from build123d import *

# Parameters (mm, degrees)
CROQUIS2_R              = 83.82
CROQUIS2_R_2            = 80.01
SALIENTE_EXTRUIR1_DEPTH = 81.28
CROQUIS4_R              = 80.01
CROQUIS4_R_2            = 76.454
SALIENTE_EXTRUIR2_DEPTH = 4.572


with BuildPart() as part:
    # Croquis2 → Saliente-Extruir1 (new body)
    with BuildSketch(Plane(origin=(0, 0, 0), x_dir=(1, 0, 0), z_dir=(0, 1, 0))):
        with Locations(Location((0, 0, 0), (0, 0, 270))):
            Circle(CROQUIS2_R)
        with Locations(Location((0, 0, 0), (0, 0, 270))):
            Circle(CROQUIS2_R_2, mode=Mode.SUBTRACT)
    extrude(amount=-SALIENTE_EXTRUIR1_DEPTH)

    # Croquis4 → Saliente-Extruir2 (add)
    with BuildSketch(Plane(origin=(0, -47.752, 0), x_dir=(1, 0, 0), z_dir=(0, 1, 0))):
        with Locations(Location((0, 0, 0), (0, 0, 270))):
            Circle(CROQUIS4_R)
        with Locations(Location((0, 0, 0), (0, 0, 270))):
            Circle(CROQUIS4_R_2, mode=Mode.SUBTRACT)
    extrude(amount=-SALIENTE_EXTRUIR2_DEPTH)


solid = part.part
Verification items for the finished model (mm, model axes). A direction names the side the tool comes from. Give positions to 0.01 mm unless a question says otherwise; leave off trailing zeros. Write each loop counter-clockwise with the first axis right and the second up, starting at its lowest first coordinate (ties: lowest second). Pieces come first, ordered by that corner, then holes. Notation, with made-up numbers: M 63.25,-30 L 85.25,-30 A17 ccw 85.25,2 Z; hole C 78,84.25 d9. An arc over 180 degrees is marked long. Put each result on its own line as item: value. Start each with the question number.
1. Section check A-A (z = 0). Record the cut outline in (x, y), and give its area (3 significant figures).
2. Section check B-B (x = 0). Record the cut outline in (y, z).
3. Scan lines: line 1 along X through (y, z) = (-33.5, 0); line 2 along X through (y, z) = (-49, 0); line 3 along Z through (x, y) = (7, -61.5). Record each from-to range of solid material in increasing order. Write a range as [from, to].
4. Draft check along Z on faces 1 (the face through (24.033, -23.542, 76.315)), 2 (the face through (70.68, -40.07, 45.06)), 3 (the face through (-74, 0, 31)). Enter one of: +Z half, -Z half, draft (parallel to the pull), parting line (faces both ways), or undercut.
5. Go/stop test with flat-tipped pins: pin 1 Ø5 at (y, z) = (-31, 44) entering from +X; pin 2 Ø6 at (x, y) = (49, -33.5) entering from -Z; pin 3 Ø8 at (y, z) = (-34, 38) entering from -X. Record where each tip stops, or that it passes through.
6. Set-up check for faces 4 (the face through (-41, -47.752, 65)), 5 (the face through (-74, -81.28, 31)), 6 (the face through (-41, -52.324, 65)): record each of +Z, -Z, +X, -X, +Y, -Y from which the full face is reachable in a straight line by a thin tool's end or side.
7. Section check C-C (y = -14). Record the cut outline in (x, z), and give its area (3 significant figures).
Answer list:
1. outline: M -83.82,-81.28 L -80.01,-81.28 L -80.01,-52.32 L -76.45,-52.32 L -76.45,-47.75 L -80.01,-47.75 L -80.01,0 L -83.82,0 Z; M 76.45,-52.32 L 80.01,-52.32 L 80.01,-81.28 L 83.82,-81.28 L 83.82,0 L 80.01,0 L 80.01,-47.75 L 76.45,-47.75 Z
1. area: 652 mm2
2. outline: M -81.28,-83.82 L 0,-83.82 L 0,-80.01 L -47.75,-80.01 L -47.75,-76.45 L -52.32,-76.45 L -52.32,-80.01 L -81.28,-80.01 Z; M -81.28,80.01 L -52.32,80.01 L -52.32,76.45 L -47.75,76.45 L -47.75,80.01 L 0,80.01 L 0,83.82 L -81.28,83.82 Z
3. line 1: [-83.82, -80.01], [80.01, 83.82]
3. line 2: [-83.82, -76.45], [76.45, 83.82]
3. line 3: [-83.53, -79.7], [79.7, 83.53]
4. face 1: undercut
4. face 2: parting line
4. face 3: draft
5. pin 1: x = 72.83
5. pin 2: z = -70.07
5. pin 3: x = -76.61
6. face 4: +Y
6. face 5: +Z, -Z, +X, -X, -Y
6. face 6: -Y
7. outline: C 0,0 d167.64; hole C 0,0 d160.02
7. area: 1,960 mm2
